```python
from build123d import *

# Parameters (mm, degrees)
F0_W     = 79.756
F0_H     = 101.6
F1_DEPTH = 1.27
F2_R     = 3.81
F3_W     = 72.136
F3_H     = 93.98
F4_DEPTH = 1.27


with BuildPart() as f1:
    # F0 (on Front) → F1 (new body, symmetric)
    with BuildSketch(Plane.XZ):
        Rectangle(F0_W, F0_H)
    extrude(amount=F1_DEPTH, both=True)

    # F2
    f2_edges = [f1.edges().sort_by_distance(p)[0] for p in [
        (-39.878, 0, 50.8),
        (39.878, 0, 50.8),
        (39.878, 0, -50.8),
        (-39.878, 0, -50.8),
    ]]
    fillet(f2_edges, radius=F2_R)

    # F3 (on face) → F4 (cut)
    with BuildSketch(Plane.XZ.offset(1.27)):
        Rectangle(F3_W, F3_H)
    extrude(amount=-F4_DEPTH, mode=Mode.SUBTRACT)


solid = f1.part
```
Geometry check sheet. Reference: the model listing, model coordinates, mm. Give positions to 0.01 mm unless a question says otherwise; leave off trailing zeros. Loops run counter-clockwise (first coordinate to the right, second up) from the corner with the lowest first, then second, coordinate; pieces in that order, holes last. Notation, with made-up numbers: M 82,-34 L 88,-34 A9 cw 88,-17 Z; hole C 73.5,31 d7. An arc over 180 degrees is marked long. Answer as CSV lines item,"result".
Item 1: Cross-section at C-C on z = 30. Record the cut outline in (x, y).
Values:
outline,"M -39.88,-1.27 L -36.07,-1.27 L -36.07,0 L 36.07,0 L 36.07,-1.27 L 39.88,-1.27 L 39.88,1.27 L -39.88,1.27 Z"
Item 2: Material ranges on line 1 (Z direction, x = 35.5, y = -0.3); line 2 (X direction, y = -0.25, z = -13); line 3 (Y direction, x = -17.5, z = -20.5), recorded low to high.
Values:
line 1,"z = -50.8 to -46.99, 46.99 to 50.8"
line 2,"x = -39.88 to -36.07, 36.07 to 39.88"
line 3,"y = 0 to 1.27"
Item 3: Depth check by flat-ended pin: P1, Ø10, axis at x = 26, z = 16, coming from the -Y side. Enter the tip coordinate at first touch or a pass-through.
Values:
P1,"stops at y = 0"
Item 4: Release check for a two-part mould opening along X. For faces 1 (the cylindrical face through (38.792, -0.018, -49.654)), 2 (the flat face through (-1, 1.27, 1)), 3 (the flat face through (-1, 0, 1)) record: pulls with the +X half, pulls with the -X half, needs draft (parallel to the pull), parting line crosses it, or undercut.
Values:
face 1,"pulls with the +X half"
face 2,"needs draft"
face 3,"undercut"
Item 5: Cross-section at A-A on y = -0.4. Record the cut outline in (x, z), and give its area (3 significant figures).
Values:
outline,"M -39.88,-46.99 A3.81 ccw -36.07,-50.8 L 36.07,-50.8 A3.81 ccw 39.88,-46.99 L 39.88,46.99 A3.81 ccw 36.07,50.8 L -36.07,50.8 A3.81 ccw -39.88,46.99 Z; hole M -36.07,-46.99 L 36.07,-46.99 L 36.07,46.99 L -36.07,46.99 Z"
area,"1,310 mm²"
Item 6: Cross-section at B-B on x = 21. Record the cut outline in (y, z).
Values:
outline,"M -1.27,-50.8 L 1.27,-50.8 L 1.27,50.8 L -1.27,50.8 L -1.27,46.99 L 0,46.99 L 0,-46.99 L -1.27,-46.99 Z"
